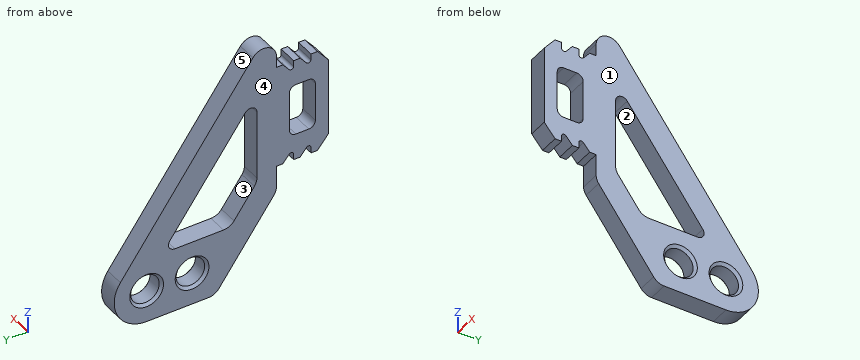
Autodesk Inventor part; units mm, degrees
ref_plane "Work Plane1" through (0, -4, -8) normal (0, 0, -1) x (-1, 0, 0)
ref_plane "YZ Plane" through (0, 0, 0) normal (1, 0, 0) x (0, 1, 0)
ref_plane "XZ Plane" through (0, 0, 0) normal (0, 1, 0) x (-1, 0, 0)
sketch "Sketch1" plane through (0, 0, 0) normal (1, 0, 0) x (0, 1, 0)
  line L0 (0, 0) -> (12.0218, -16.5295)
  line L1 (10, -20.5) -> (4.7274, -20.5)
  line L2 (0, -14) -> (4.7274, -20.5)
  line L3 (0, 0) -> (0, -4)
  line L4 (0, -4) -> (-4, -4)
  line L5 (-4, -4) -> (-4, -12)
  line L6 (-4, -12) -> (0, -12)
  line L7 (0, -12) -> (0, -14)
  arc A0 (10, -20.5) -> (12.0218, -16.5295) centre (10, -18) ccw
  point P0 (14.9095, -20.5)
  point P1 (6.5, -18)
  dimension "d26" = 8
  dimension "d31" = 4
  dimension "d32" = 2
  dimension "d43" = 2.5
  dimension "d45" = 10
  dimension "d64" = 3.5
  dimension "d65" = 4
  dimension "d78" = 18
extrude "Extrusion1" add sketch "Sketch1" along normal blind 1.5
hole "Hole3" at (0, 10, -18) at (0, 6.5, -18) direction (1, 0, 0) diameter 2.2 end through all
fillet "Fillet3" radius 1 3 edges at (0.75, 0, 0) (0.75, 4.7274, -20.5) (0.75, 0, -14)
chamfer "Chamfer2" distance 0.2 angle 45 4 edges at (1.5, 6.5, -19.1) (1.5, 10, -19.1) (0, 6.5, -19.1) (0, 10, -19.1)
ref_plane "Work Plane1" through (0, -4, -8) normal (0, 0, -1) x (-1, 0, 0)
sketch "Sketch4" plane through (1.5, 0, 0) normal (1, 0, 0) x (0, 0, -1)
  arc A0 (2.4869, 1.8087) -> (3.0751, 0) centre (3.0751, 1) ccw
  line L0 (3.0751, 0) -> (4, 0)
  line L1 (4, 0) -> (4, -4)
  line L2 (4, -4) -> (12, -4)
  line L3 (12, -4) -> (12, 0)
  line L4 (12, 0) -> (13.6748, 0)
  line L5 (14.263, 0.1913) -> (20.0882, 4.4279)
  line L6 (20.5, 5.2366) -> (20.5, 10)
  arc A1 (20.5, 10) -> (16.5295, 12.0218) centre (18, 10) ccw
  line L7 (16.5295, 12.0218) -> (2.4869, 1.8087)
  circle A2 centre (18, 10) radius 1.3
  line L8 (4, 0) -> (12, 0)
  line L9 (12, -4) -> (4, -4)
  line L10 (5, -4) -> (4, -3.1667)
  line L11 (4, -4) -> (4, 0)
  line L12 (4, -2.6667) -> (5, -2.6667)
  line L13 (5, -2.6667) -> (4, -1.8333)
  line L14 (4, -1.3333) -> (5, -1.3333)
  line L15 (5, -1.3333) -> (4, -0.5)
  line L16 (4, -0.5) -> (4, 0)
  line L17 (4, -0.5) -> (4, -1.3333)
  line L18 (4, -1.8333) -> (4, -2.6667)
  line L19 (4, -3.1667) -> (4, -4)
  line L20 (4, -4) -> (5, -4)
  arc A3 (13.6748, 0) -> (14.263, 0.1913) centre (13.6748, 1) ccw
  arc A4 (20.0882, 4.4279) -> (20.5, 5.2366) centre (19.5, 5.2366) ccw
  point P0 (0, 0)
  dimension "d57" = 1
  dimension "d58" = 0.5
  dimension "d59" = 0.5
  dimension "d60" = 0.5
extrude "Extrusion2" cut sketch "Sketch4" against normal through all contours L15 L14 L1 | L13 L12 L1 | L2 L1 L10
mirror "Mirror1" about plane through (0, -4, -8) normal (0, 0, -1) of "Extrusion2"
fillet "Fillet4" radius 0.2 4 edges at (0.75, -1.3333, -11) (0.75, -2.6667, -11) (0.75, -1.3333, -5) (0.75, -2.6667, -5)
sketch "Sketch5" plane through (1.5, 0, 0) normal (1, 0, 0) x (0, 0, -1)
  line L0 (5.4627, 1.5) -> (12.6621, 1.5)
  line L1 (12.6621, 1.5) -> (15.5, 3.564)
  line L2 (15.5, 3.564) -> (15.5, 8.8)
  line L3 (15.5, 8.8) -> (5.4627, 1.5)
  line L4 (16.5295, 12.0218) -> (2.4869, 1.8087)
  circle A0 centre (18, 6.5) radius 1.3
  line L5 (14.263, 0.1913) -> (20.0882, 4.4279)
  line L6 (12, 0) -> (13.6748, 0)
  line L7 (6, -1) -> (10, -1)
  line L8 (10, -1) -> (10, -3)
  line L9 (10, -3) -> (6, -3)
  line L10 (6, -3) -> (6, -1)
  line L11 (5, -4) -> (11, -4)
  line L12 (12, -0.5) -> (12, 0)
  line L13 (4, 0) -> (4, -0.5)
  point P0 (0, 0)
  point P1 (14, 0)
  point P2 (21.5, 5.144)
  dimension "d66" = 2.5
  dimension "d67" = 2
  dimension "d68" = 2
  dimension "d69" = 1.5
  dimension "d74" = 1
  dimension "d75" = 1
  dimension "d76" = 2
  dimension "d77" = 2
extrude "Extrusion3" cut sketch "Sketch5" against normal through all contours L3 L2 L1 L0 | L7 L8 L9 L10
fillet "Fillet5" radius 0.5 6 edges at (0.75, 1.5, -5.4627) (0.75, 8.8, -15.5) (0.75, -3, -6) (0.75, -1, -6) (0.75, -1, -10) (0.75, -3, -10)
fillet "Fillet5" radius 1 2 edges at (0.75, 3.564, -15.5) (0.75, 1.5, -12.6621)
equation "\"d46\" = hole_diameter"
equation "\"d59\" = d58"
equation "\"d60\" = d58"
equation "\"d68\" = d67"
equation "\"d77\" = d76"
equation "\"d1\" = d0"
equation "\"d21\" = d1"
equation "\"hole_diameter\" = 2.2"
properties part number "M2_LINKAGE" material "ABS Plastic"
Geometry check sheet. Reference: the model listing, model coordinates, mm. Face numbers are marked on the shaded views. A direction names the side the tool comes from. Give positions to 0.01 mm unless a question says otherwise; leave off trailing zeros. Order: outer loops, then holes, each group sorted by start corner. A loop starts at its lowest first (then second) coordinate and runs counter-clockwise, first axis right, second up. Notation, with made-up numbers: (19.5, 12.5) - (32.5, 12.5) arc R6 ccw to (32.5, 22.5) - close; hole circle Ø4 at (-11, -18.5). An arc over 180 degrees is marked (long way). Answer as a JSON object with one key per item and string values.
(1) Cross-section at A-A (z = -10.75). Record the cut outline in (x, y), then the cut area to 3 significant figures.
Report:
{"outline": "(0, -4) - (1.5, -4) - (1.5, 1.5) - (0, 1.5) - close; (0, 5.35) - (1.5, 5.35) - (1.5, 7.82) - (0, 7.82) - close", "area": "12.0 mm^2"}
(2) Draft check along Y on the marked faces 3, 4 and 5. Enter one of: released by +Y, released by -Y, zero draft, split by the parting line, or undercut.
Report:
{"face 3": "undercut", "face 4": "zero draft", "face 5": "released by +Y"}
(3) Cross-section at C-C (z = -18). Record the cut outline in (x, y), then the cut area to 3 significant figures.
Report:
{"outline": "(0, 2.91) - (1.5, 2.91) - (1.5, 5.2) - (1.3, 5.4) - (0.2, 5.4) - (0, 5.2) - close; (0, 7.8) - (0.2, 7.6) - (1.3, 7.6) - (1.5, 7.8) - (1.5, 8.7) - (1.3, 8.9) - (0.2, 8.9) - (0, 8.7) - close; (0, 11.3) - (0.2, 11.1) - (1.3, 11.1) - (1.5, 11.3) - (1.5, 12.5) - (0, 12.5) - close", "area": "7.63 mm^2"}
(4) Cross-section at D-D (y = 6.5). Record the cut outline in (x, z), then the cut area to 3 significant figures.
Report:
{"outline": "(0, -20.5) - (1.5, -20.5) - (1.5, -19.3) - (1.3, -19.1) - (0.2, -19.1) - (0, -19.3) - close; (0, -16.7) - (0.2, -16.9) - (1.3, -16.9) - (1.5, -16.7) - (1.5, -15.5) - (0, -15.5) - close; (0, -12.34) - (1.5, -12.34) - (1.5, -8.94) - (0, -8.94) - close", "area": "9.22 mm^2"}
(5) Depth check by flat-ended pin: pin 1 Ø0.5 at (x, y) = (1, -2) entering from -Z; pin 2 Ø1 at (y, z) = (8, -7) entering from +X; pin 3 Ø0.5 at (x, z) = (1, -4) entering from +Y. Enter the tip coordinate at first touch or a pass-through.
Report:
{"pin 1": "z = -12", "pin 2": "through", "pin 3": "y = 3.09"}
(6) Tool access check on the marked faces 1 and 2. Record the directions out of +Z, -Z, +X, -X, +Y, -Y that give a thin tool (end or side, any length) a straight path to the whole face; none if there is none.
Report:
{"face 1": "+Z, -Z, +X, +Y, -Y", "face 2": "+X, -X"}
(7) Material ranges on line 1 (Z direction, x = 0.3, y = -1.5); line 2 (Z direction, x = 0.5, y = 6.5); line 3 (Y direction, x = 0.7, z = -18), recorded low to high.
Report:
{"line 1": "-12 to -10, -6 to -4", "line 2": "-20.5 to -19.1, -16.9 to -15.5, -12.34 to -8.94", "line 3": "2.91 to 5.4, 7.6 to 8.9, 11.1 to 12.5"}
(8) Cross-section at B-B (y = 3.5). Record the cut outline in (x, z).
Report:
{"outline": "(0, -18.81) - (1.5, -18.81) - (1.5, -15.32) - (0, -15.32) - close; (0, -8.21) - (1.5, -8.21) - (1.5, -4.81) - (0, -4.81) - close"}
